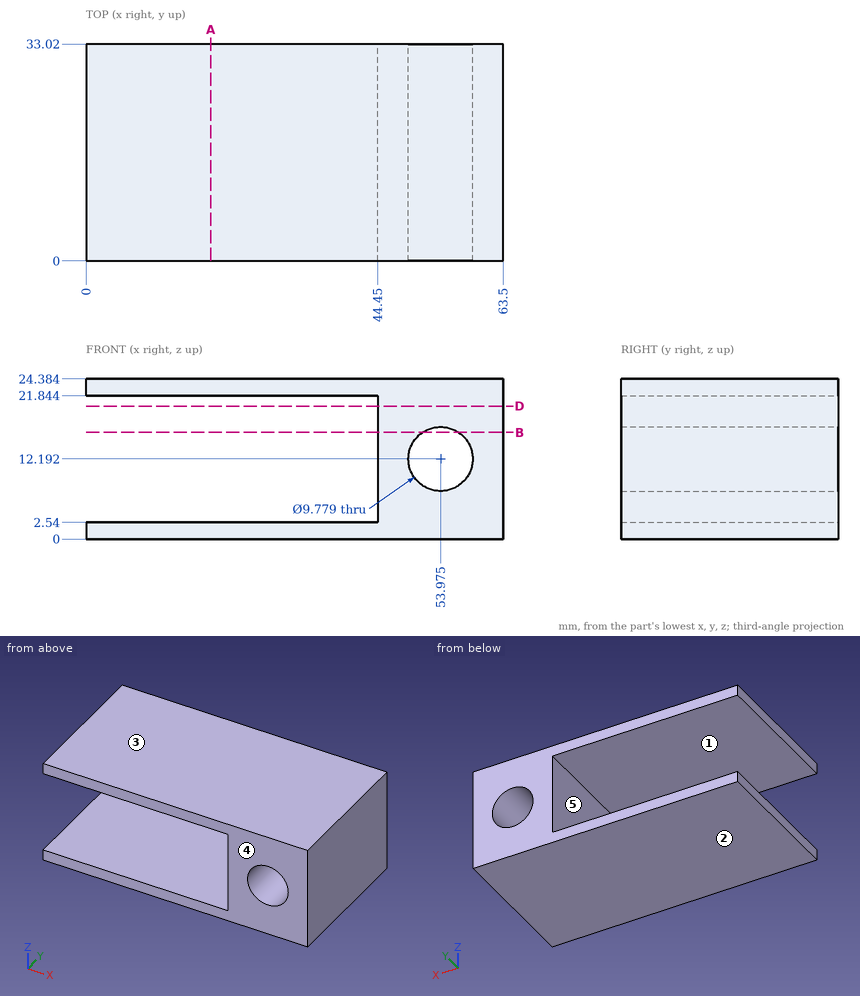
Geometry: see drawing. Coordinates: mm, zero at the bounding-box minimum. A direction names the side the tool comes from. Give positions to 0.01 mm unless a question says otherwise; leave off trailing zeros. Write each loop counter-clockwise with the first axis right and the second up, starting at its lowest first coordinate (ties: lowest second). Pieces come first, ordered by that corner, then holes. Notation, with made-up numbers: (85.25, 45) - (111.25, 45) arc R13 ccw to (111.25, 70) - close; hole circle Ø5 at (83.5, 84.5). An arc over 180 degrees is marked (long way). Return JSON: item names as keys, results as strings. Group by question number.
1) Line query: line 1 (Z direction, x = 42.5, y = 16); line 2 (X direction, y = 19.5, z = 12.25); line 3 (X direction, y = 20, z = 19.5). Output: solid intervals per line, ascending.
2) Section D-D on z = 20.25. Return the cut outline in (x, y), plus the area to 3 significant figures.
3) Set-up query: the marked faces 1 and 2. Return all of +Z, -Z, +X, -X, +Y, -Y with unobstructed straight access to the full face (end or side cutting, diameter ignored); none if empty.
4) Section A-A on x = 19. Return the cut outline in (y, z).
5) Mould query, pull axis Z, two halves, no side actions, for the marked faces 3, 4 and 5. Classes: released by +Z, released by -Z, zero draft, split by the parting line, or undercut.
6) First-contact query: P1, Ø5, axis at y = 7, z = 10.5, coming from the -X side. Flat tip, straight axial feed; report the tip coordinate or a pass-through.
7) Section B-B on z = 16.25. Return the cut outline in (x, y).
Filled in:
{
 "1": {"line 1": "z = 0 to 2.54, 21.84 to 24.38", "line 2": "x = 44.45 to 49.09, 58.86 to 63.5", "line 3": "x = 44.45 to 63.5"},
 "2": {"outline": "(44.45, 0) - (63.5, 0) - (63.5, 33.02) - (44.45, 33.02) - close", "area": "629 mm^2"},
 "3": {"face 1": "-X, +Y, -Y", "face 2": "-Z, +X, -X, +Y, -Y"},
 "4": {"outline": "(0, 0) - (33.02, 0) - (33.02, 2.54) - (0, 2.54) - close; (0, 21.84) - (33.02, 21.84) - (33.02, 24.38) - (0, 24.38) - close"},
 "5": {"face 3": "released by +Z", "face 4": "zero draft", "face 5": "undercut"},
 "6": {"P1": "stops at x = 44.45"},
 "7": {"outline": "(44.45, 0) - (51.25, 0) - (51.25, 33.02) - (44.45, 33.02) - close; (56.7, 0) - (63.5, 0) - (63.5, 33.02) - (56.7, 33.02) - close"}
}
